CAD build for the part. Positions are in the model's coordinates, mm. A direction names the side the tool comes from. Coordinates: 2 decimals unless noted, no trailing zeros. Loops run counter-clockwise (first coordinate to the right, second up) from the corner with the lowest first, then second, coordinate; pieces in that order, holes last.
1) Saw through at A-A, the plane x = 22.5. Write the cut outline in (y, z).
2) Wall check: line 1 along Y through (x, z) = (-0.5, 1.2); line 2 along Y through (x, z) = (24.5, 1.7); line 3 along Y through (x, z) = (-23, 0.9). Give the ranges that are in metal, low to high.
3) Saw through at B-B, the plane z = 1.3. Write the cut outline in (x, y), and give its area (3 significant figures).
4) Saw through at C-C, the plane y = 6.75. Write the cut outline in (x, z), and give its area (3 significant figures).
5) Two-plate mould, pull along Y, no slides. Class faces 1 (the cylindrical face through (-19.25, 3.09, 1.01)), 2 (the flat face through (26, -1.25, 1)), 3 (the flat face through (0, 13, 1)), 4 (the cylindrical face through (-25.463, -7.344, 0.986)): +Y half, -Y half, draft (parallel to the pull), parting line (faces both ways), or undercut.
6) Which spindle directions (+Z, -Z, +X, -X, +Y, -Y) get a long thin tool onto all of the face, cutting with end or side? Do faces 5 (the flat face through (-26, 7.25, 1)), 6 (the flat face through (26, 7.25, 1)), 7 (the flat face through (-8, 14, 1)), 8 (the flat face through (0, -9.642, 1)). Say none if no direction does.
7) Pin check, flat tips, straight feed: pin 1 Ø0.6 at (x, z) = (-25, 1) entering from -Y; pin 2 Ø0.6 at (x, z) = (-25.5, 1.5) entering from +Y; pin 3 Ø0.6 at (x, z) = (25, 1) entering from +Y. Stop position of each tip, or through.
8) Saw through at D-D, the plane x = 1. Write the cut outline in (y, z).
```python
from build123d import *

# Parameters (mm, degrees)
SKETCH_1_R          = 3.25
EXTRUDE_1_DEPTH     = 2
CUT_EXTRUDE_2_DEPTH = 2


with BuildPart() as part:
    # Эскиз1 → Бобышка-Вытянуть1 (new body)
    with BuildSketch(Plane.XY):
        with BuildLine():
            Line((-8, 15.642410702), (-20, 15.642410702))
            ThreePointArc((-20, 15.642410702), (-25.404000432, 13.404000432), (-27.642410702, 8))
            Line((-27.642410702, 8), (-27.642410702, -2))
            ThreePointArc((-27.642410702, -2), (-25.404000432, -7.404000432), (-20, -9.642410702))
            Line((-20, -9.642410702), (20, -9.642410702))
            ThreePointArc((20, -9.642410702), (25.404000432, -7.404000432), (27.642410702, -2))
            Line((27.642410702, -2), (27.642410702, 8))
            ThreePointArc((27.642410702, 8), (25.404000432, 13.404000432), (20, 15.642410702))
            Line((20, 15.642410702), (8, 15.642410702))
            Line((8, 15.642410702), (8, 13))
            Line((8, 13), (-8, 13))
            Line((-8, 13), (-8, 15.642410702))
        make_face()
        with Locations((23.5, 3)):
            Circle(SKETCH_1_R, mode=Mode.SUBTRACT)
        with Locations((-23.5, 3)):
            Circle(SKETCH_1_R, mode=Mode.SUBTRACT)
    extrude(amount=EXTRUDE_1_DEPTH)

    # Эскиз3 → Вырез-Вытянуть2 (cut)
    with BuildSketch(Plane.XY.offset(2)):
        with BuildLine():
            Line((-23.5, -1.25), (-30.303484741, -1.25))
            ThreePointArc((-30.303484741, -1.25), (-34.553484741, 3), (-30.303484741, 7.25))
            Line((-30.303484741, 7.25), (-23.5, 7.25))
            ThreePointArc((-23.5, 7.25), (-19.25, 3), (-23.5, -1.25))
        make_face()
        with BuildLine():
            Line((23.5, -1.25), (30.303484741, -1.25))
            ThreePointArc((30.303484741, -1.25), (34.553484741, 3), (30.303484741, 7.25))
            Line((30.303484741, 7.25), (23.5, 7.25))
            ThreePointArc((23.5, 7.25), (19.25, 3), (23.5, -1.25))
        make_face()
    extrude(amount=-CUT_EXTRUDE_2_DEPTH, mode=Mode.SUBTRACT)


solid = part.part
```
Data:
1. outline: (-9.22, 0) - (-1.13, 0) - (-1.13, 2) - (-9.22, 2) - close; (7.13, 0) - (15.22, 0) - (15.22, 2) - (7.13, 2) - close
2. line 1: y = -9.64 to 13
2. line 2: y = -8.18 to -1.25, 7.25 to 14.18
2. line 3: y = -9.03 to -1.22, 7.22 to 15.03
3. outline: (-27.64, -2) arc R7.64 ccw to (-20, -9.64) - (20, -9.64) arc R7.64 ccw to (27.64, -2) - (27.64, -1.25) - (23.5, -1.25) arc R4.25 cw to (23.5, 7.25) - (27.64, 7.25) - (27.64, 8) arc R7.64 ccw to (20, 15.64) - (8, 15.64) - (8, 13) - (-8, 13) - (-8, 15.64) - (-20, 15.64) arc R7.64 ccw to (-27.64, 8) - (-27.64, 7.25) - (-23.5, 7.25) arc R4.25 cw to (-23.5, -1.25) - (-27.64, -1.25) - close
3. area: 1,180 mm2
4. outline: (-21.5, 0) - (21.5, 0) - (21.5, 2) - (-21.5, 2) - close
4. area: 86.0 mm2
5. face 1: undercut
5. face 2: undercut
5. face 3: +Y half
5. face 4: -Y half
6. face 5: +Z, -Z, -X
6. face 6: +Z, -Z, +X
6. face 7: +Z, -Z, +Y
6. face 8: +Z, -Z, +X, -X, -Y
7. pin 1: stops at y = -8.03
7. pin 2: stops at y = 13.6
7. pin 3: stops at y = 14.03
8. outline: (-9.64, 0) - (13, 0) - (13, 2) - (-9.64, 2) - close
